```python
from build123d import *

# Parameters (mm, degrees)
F0_R     = 25
F1_DEPTH = 25


with BuildPart() as f1:
    # F0 (on Front) → F1 (new body)
    with BuildSketch(Plane.XZ):
        with BuildLine():
            ThreePointArc((-17.005196, 20.183328), (-16.891213, 21.625071), (-16.853183, 23.070812))
            ThreePointArc((-16.853183, 23.070812), (-16.854895, 23.37759), (-16.860028, 23.68433))
            ThreePointArc((-16.860028, 23.68433), (-71.829573, 24.21011), (-17.005196, 20.183328))
        make_face()
        with Locations((-44.353183, 23.070812)):
            Circle(F0_R, mode=Mode.SUBTRACT)
        with BuildLine():
            ThreePointArc((-16.860028, 23.68433), (-16.854895, 23.37759), (-16.853183, 23.070812))
            ThreePointArc((-16.853183, 23.070812), (-16.891213, 21.625071), (-17.005196, 20.183328))
            ThreePointArc((-17.005196, 20.183328), (-2.472507, 27.848748), (11.767841, 19.653005))
            ThreePointArc((11.767841, 19.653005), (11.585381, 21.770557), (11.567004, 23.895875))
            ThreePointArc((11.567004, 23.895875), (-2.710738, 32.420641), (-16.860028, 23.68433))
        make_face()
        with BuildLine():
            ThreePointArc((66.554625, 23.070812), (39.467203, 50.567717), (11.567004, 23.895875))
            ThreePointArc((11.567004, 23.895875), (11.585381, 21.770557), (11.767841, 19.653005))
            ThreePointArc((11.767841, 19.653005), (40.766851, -4.375832), (66.554625, 23.070812))
        make_face()
        with Locations((39.054625, 23.070812)):
            Circle(F0_R, mode=Mode.SUBTRACT)
    extrude(amount=F1_DEPTH)


solid = f1.part
```
CAD build for the part. Positions are in the model's coordinates, mm. Give positions to 0.01 mm unless a question says otherwise; leave off trailing zeros. Loops run counter-clockwise (first coordinate to the right, second up) from the corner with the lowest first, then second, coordinate; pieces in that order, holes last. Notation, with made-up numbers: (10, 15) -> (37, 15) arc R29 ccw to (37, 38) -> close; hole circle Ø11 at (15.5, -0.5). An arc over 180 degrees is marked (long way). Use a Markdown table: item, result.
1. Slice it at C-C (y = -18.5). List the corners of the cut face in (x, z).
Check result:
| item | result |
|---|---|
| outline | (-17.01, 20.18) arc R17.02 cw to (11.77, 19.65) arc R27.5 ccw (long way) to (11.57, 23.9) arc R16.02 ccw to (-16.86, 23.68) arc R27.5 ccw (long way) to start; hole circle Ø50 at (-44.35, 23.07); hole circle Ø50 at (39.05, 23.07) |
2. Flat gauge pins, fed straight in: pin 1 (4 mm diameter, centred on x = 3, z = 32.5, fed in from +Y); pin 2 (4 mm diameter, centred on x = 22.5, y = -8.5, fed in from -Z); pin 3 (4 mm diameter, centred on x = -29, y = -20, fed in from -Z); pin 4 (4 mm diameter, centred on y = -19.5, z = 36, fed in from +X). Where does each tip first touch, or does it go through?
Check result:
| item | result |
|---|---|
| pin 1 | stops at y = 0 |
| pin 2 | stops at z = -0.26 |
| pin 3 | stops at z = -0.97 |
| pin 4 | stops at x = 64.29 |
3. Slice it at D-D (z = 4.5). List the corners of the cut face in (x, y), plus the area to 3 significant figures.
Check result:
| item | result |
|---|---|
| outline | (-64.64, -25) -> (-61.09, -25) -> (-61.09, 0) -> (-64.64, 0) -> close; (-27.62, -25) -> (-24.07, -25) -> (-24.07, 0) -> (-27.62, 0) -> close; (18.77, -25) -> (22.32, -25) -> (22.32, 0) -> (18.77, 0) -> close; (55.79, -25) -> (59.34, -25) -> (59.34, 0) -> (55.79, 0) -> close |
| area | 355 mm^2 |
4. Wall check: L1, parallel to X at y = -14, z = 34; L2, parallel to X at y = -8.75, z = 14.5; L3, parallel to Z at x = 38.5, y = -12.5. Give the ranges that are in metal, low to high. Write a range as [from, to].
Check result:
| item | result |
|---|---|
| L1 | x = [-69.59, -66.84], [-21.87, -19.12], [13.82, 16.57], [61.54, 64.29] |
| L2 | x = [-70.48, -67.84], [-20.87, -18.22], [12.92, 15.57], [62.54, 65.18] |
| L3 | z = [-4.42, -1.92], [48.06, 50.57] |
5. Mould opens along X. For faces 1 (the cylindrical face through (-2.47, -12.32, 32.42)), 2 (the flat face through (-8.1, 0, 27.3)) say: pulls with the +X half, pulls with the -X half, needs draft (parallel to the pull), parting line crosses it, or undercut.
Check result:
| item | result |
|---|---|
| face 1 | undercut |
| face 2 | needs draft |
6. Slice it at A-A (x = -31). List the corners of the cut face in (y, z), plus the area to 3 significant figures.
Check result:
| item | result |
|---|---|
| outline | (-25, -0.97) -> (0, -0.97) -> (0, 1.94) -> (-25, 1.94) -> close; (-25, 44.21) -> (0, 44.21) -> (0, 47.11) -> (-25, 47.11) -> close |
| area | 145 mm^2 |
7. Slice it at B-B (z = 38). List the corners of the cut face in (x, y).
Check result:
| item | result |
|---|---|
| outline | (-67.45, -25) -> (-64.41, -25) -> (-64.41, 0) -> (-67.45, 0) -> close; (-24.3, -25) -> (-21.26, -25) -> (-21.26, 0) -> (-24.3, 0) -> close; (15.96, -25) -> (19, -25) -> (19, 0) -> (15.96, 0) -> close; (59.11, -25) -> (62.15, -25) -> (62.15, 0) -> (59.11, 0) -> close |
